Read the model definition and answer for the solid it produces. Units are mm, in the model's axes. A direction names the side the tool comes from. Coordinates: 2 decimals unless noted, no trailing zeros. Loops run counter-clockwise (first coordinate to the right, second up) from the corner with the lowest first, then second, coordinate; pieces in that order, holes last.
Q1. Straight lines are drawn through the part: line 1 (Y direction, x = 2.75, z = -69); line 2 (Z direction, x = 3.5, y = -29); line 3 (Y direction, x = 6.75, z = 66). For each, find the intervals that lie inside material, in ascending order.
Q2. Flat-ended cylindrical pins translate along their axes: P1, Ø4, axis at x = 9, z = 67, coming from the -Y side; P2, Ø6.5, axis at x = 6, z = -67, coming from the +Y side; P3, Ø4, axis at x = 5, y = -13, coming from the -Z side; P4, Ø4, axis at x = 6.5, y = -30.5, coming from the +Z side. Find the tip coordinate at first contact, or state that the pin passes through.
Q3. Section A-A (y = -27) is taken. Give the vertices of the cut face in (x, z).
Q4. Section B-B (y = -19) is taken. Give the vertices of the cut face in (x, z).
Q5. Section C-C (z = 10) is taken. Give the vertices of the cut face in (x, y), then the cut area to 3 significant figures.
Q6. The mould has two halves that part along Z. Classify faces 4 (the face through (6, -25.4, -70)), 5 (the face through (6, -19, 76.2)), 6 (the face through (6, -32, -50.8)): pulls with the +Z half, pulls with the -Z half, needs draft (parallel to the pull), parting line crosses it, or undercut.
Q7. Which of the six approach directions +Z, -Z, +X, -X, +Y, -Y give full straight-line access (tool end or side, diameter ignored) to faces 1 (the face through (6, -32, 0)), 2 (the face through (6, -19, -63.5)), 3 (the face through (6, 12.7, 70))?
from build123d import *

# Parameters (mm, degrees)
SKETCH1_W           = 152.4
SKETCH1_H           = 76.2
BOSS_EXTRUDE1_DEPTH = 12.7
SKETCH2_W           = 12.7
SKETCH2_H           = 12.7
CUT_EXTRUDE1_DEPTH  = 87.135590786
SKETCH3_W           = 12.7
SKETCH3_H           = 12.7
CUT_EXTRUDE2_DEPTH  = 12.7


with BuildPart() as part:
    # Sketch1 → Boss-Extrude1 (new body)
    with BuildSketch(Plane(origin=(0, 0, 0), x_dir=(0, 0, -1), z_dir=(1, 0, 0))):
        Rectangle(SKETCH1_W, SKETCH1_H)
    extrude(amount=BOSS_EXTRUDE1_DEPTH)

    # Sketch2 → Cut-Extrude1 (cut, through all)
    with BuildSketch(Plane(origin=(12.7, 0, 0), x_dir=(0, 0, -1), z_dir=(1, 0, 0))):
        with Locations((-69.85, 19.05)):
            Rectangle(SKETCH2_W, SKETCH2_H)
        with Locations((-69.85, -6.35)):
            Rectangle(SKETCH2_W, SKETCH2_H)
        with Locations((-69.85, -31.75)):
            Rectangle(SKETCH2_W, SKETCH2_H)
        with Locations((69.85, 31.75)):
            Rectangle(SKETCH2_W, SKETCH2_H)
        with Locations((69.85, 6.35)):
            Rectangle(SKETCH2_W, SKETCH2_H)
        with Locations((69.85, -19.05)):
            Rectangle(SKETCH2_W, SKETCH2_H)
    extrude(amount=-CUT_EXTRUDE1_DEPTH, mode=Mode.SUBTRACT)

    # Sketch3 → Cut-Extrude2 (cut)
    with BuildSketch(Plane(origin=(90.45925552, -38.1, 56.334406979), x_dir=(0, 0, 1), z_dir=(0, -1, 0))):
        with Locations((-100.784406979, 84.10925552)):
            Rectangle(SKETCH3_W, SKETCH3_H)
        with Locations((-75.384406979, 84.10925552)):
            Rectangle(SKETCH3_W, SKETCH3_H)
        with Locations((-49.984406979, 84.10925552)):
            Rectangle(SKETCH3_W, SKETCH3_H)
        with Locations((-24.584406979, 84.10925552)):
            Rectangle(SKETCH3_W, SKETCH3_H)
        with Locations((0.815593021, 84.10925552)):
            Rectangle(SKETCH3_W, SKETCH3_H)
    extrude(amount=-CUT_EXTRUDE2_DEPTH, mode=Mode.SUBTRACT)


solid = part.part
Numbers:
1. line 1: y = -38.1 to -25.4, -12.7 to 0, 12.7 to 25.4
1. line 2: z = -76.2 to -50.8, -38.1 to -25.4, -12.7 to 0, 12.7 to 25.4, 38.1 to 50.8
1. line 3: y = -25.4 to -12.7, 0 to 12.7, 25.4 to 38.1
2. P1: stops at y = -25.4
2. P2: stops at y = 25.4
2. P3: stops at z = -76.2
2. P4: stops at z = 50.8
3. outline: (0, -76.2) - (12.7, -76.2) - (12.7, -50.8) - (0, -50.8) - close; (0, -38.1) - (12.7, -38.1) - (12.7, -25.4) - (0, -25.4) - close; (0, -12.7) - (12.7, -12.7) - (12.7, 0) - (0, 0) - close; (0, 12.7) - (12.7, 12.7) - (12.7, 25.4) - (0, 25.4) - close; (0, 38.1) - (12.7, 38.1) - (12.7, 50.8) - (0, 50.8) - close
4. outline: (0, -63.5) - (12.7, -63.5) - (12.7, 76.2) - (0, 76.2) - close
5. outline: (0, -25.4) - (12.7, -25.4) - (12.7, 38.1) - (0, 38.1) - close
5. area: 806 mm2
6. face 4: needs draft
6. face 5: pulls with the +Z half
6. face 6: undercut
7. face 1: +X, -X, -Y
7. face 2: -Z, +X, -X
7. face 3: +Z, +X, -X
